Source: CAD feature listing. Evaluate the final solid. Frame: model axes, mm. Face numbers are marked on the shaded views. A direction names the side the tool comes from. Give positions to 0.01 mm unless a question says otherwise; leave off trailing zeros. Write each loop counter-clockwise with the first axis right and the second up, starting at its lowest first coordinate (ties: lowest second). Pieces come first, ordered by that corner, then holes. Notation, with made-up numbers: (-5, 74) -> (34, 74) arc R20 ccw to (34, 96) -> close; hole circle Ø3 at (35.25, 15.25). An arc over 180 degrees is marked (long way). Write item = value, one per line.
from build123d import *

# Parameters (mm, degrees)
SALIENTE_EXTRUIR1_DEPTH = 10
CROQUIS5_R              = 16.5
CORTAR_EXTRUIR4_DEPTH   = 3
CROQUIS4_R              = 1.5
CORTAR_EXTRUIR8_DEPTH   = 126.015998976
CROQUIS6_W              = 60
CROQUIS6_H              = 90.5
SALIENTE_EXTRUIR2_DEPTH = 5
CROQUIS7_R              = 11.25
CROQUIS7_R_2            = 1.5
CORTAR_EXTRUIR9_DEPTH   = 10
SALIENTE_EXTRUIR3_DEPTH = 46
CROQUIS10_W             = 5
CROQUIS10_H             = 5
CORTAR_EXTRUIR11_DEPTH  = 5
CROQUIS11_R             = 1.5
CORTAR_EXTRUIR12_DEPTH  = 168.751304019
CROQUIS13_W             = 43
CROQUIS13_H             = 43
CORTAR_EXTRUIR13_DEPTH  = 2
CROQUIS16_R             = 1
CORTAR_EXTRUIR14_DEPTH  = 10
NERVIO1_REACH           = 159.779
CROQUIS17_WALL_W        = 345.058235512
CROQUIS17_WALL_H        = 10
REDONDEO2_R             = 5
CROQUIS18_W             = 13
CROQUIS18_H             = 12
CORTAR_EXTRUIR15_DEPTH  = 10


with BuildPart() as part:
    # Croquis1 → Saliente-Extruir1 (new body)
    with BuildSketch(Plane.XY):
        with BuildLine():
            Line((-30, -95), (-30, -115))
            Line((-30, -115), (30, -115))
            Line((30, -115), (30, -95))
            ThreePointArc((30, -95), (35.193890367, -54.576427951), (45.544194453, -15.156726282))
            ThreePointArc((45.544194453, -15.156726282), (0, 48), (-45.544194453, -15.156726282))
            ThreePointArc((-45.544194453, -15.156726282), (-35.193890367, -54.576427951), (-30, -95))
        make_face()
    extrude(amount=SALIENTE_EXTRUIR1_DEPTH)

    # Croquis5 → Cortar-Extruir4 (cut)
    with BuildSketch(Plane.XY.offset(10)):
        Circle(CROQUIS5_R)
    extrude(amount=-CORTAR_EXTRUIR4_DEPTH, mode=Mode.SUBTRACT)

    # Croquis4 → Cortar-Extruir8 (cut, through all)
    with BuildSketch(Plane(origin=(0, 0, 10), x_dir=(-1, 0, 0), z_dir=(0, 0, 1))):
        with Locations(Location((0, 12, 0), (0, 0, 180))):
            Circle(CROQUIS4_R)
        with Locations(Location((12, 0, 0), (0, 0, 180))):
            Circle(CROQUIS4_R)
        with Locations(Location((0, -12, 0), (0, 0, 180))):
            Circle(CROQUIS4_R)
        with Locations(Location((-12, 0, 0), (0, 0, 180))):
            Circle(CROQUIS4_R)
    extrude(amount=-CORTAR_EXTRUIR8_DEPTH, mode=Mode.SUBTRACT)

    # Croquis6 → Saliente-Extruir2 (add)
    with BuildSketch(Plane.XZ.offset(115)):
        with Locations((0, 45.25)):
            Rectangle(CROQUIS6_W, CROQUIS6_H)
    extrude(amount=SALIENTE_EXTRUIR2_DEPTH)

    # Croquis7 → Cortar-Extruir9 (cut)
    with BuildSketch(Plane.XZ.offset(120)):
        with Locations(Location((0, 64, 0), (0, 0, 270))):
            Circle(CROQUIS7_R)
        with Locations(Location((-15.5, 79.5, 0), (0, 0, 270))):
            Circle(CROQUIS7_R_2)
        with Locations(Location((15.5, 79.5, 0), (0, 0, 270))):
            Circle(CROQUIS7_R_2)
        with Locations(Location((15.5, 48.5, 0), (0, 0, 270))):
            Circle(CROQUIS7_R_2)
        with Locations(Location((-15.5, 48.5, 0), (0, 0, 270))):
            Circle(CROQUIS7_R_2)
    extrude(amount=-CORTAR_EXTRUIR9_DEPTH, mode=Mode.SUBTRACT)

    # Croquis8 → Saliente-Extruir3 (add)
    with BuildSketch(Plane(origin=(0, -115, 0), x_dir=(1, 0, 0), z_dir=(0, 1, 0))):
        Polygon((-21.5, -42.5), (21.5, -42.5), (21.5, -90.5), (26.5, -90.5), (26.5, -37.5), (-26.5, -37.5), (-26.5, -90.5), (-21.5, -90.5), align=None)
    extrude(amount=SALIENTE_EXTRUIR3_DEPTH)

    # Croquis10 → Cortar-Extruir11 (cut)
    with BuildSketch(Plane.XY.offset(90.5)):
        with Locations((24, -107.5)):
            Rectangle(CROQUIS10_W, CROQUIS10_H)
        with Locations((-24, -107.5)):
            Rectangle(CROQUIS10_W, CROQUIS10_H)
        with Locations((-24, -97.5)):
            Rectangle(CROQUIS10_W, CROQUIS10_H)
        with Locations((24, -97.5)):
            Rectangle(CROQUIS10_W, CROQUIS10_H)
        with Locations((-24, -87.5)):
            Rectangle(CROQUIS10_W, CROQUIS10_H)
        with Locations((24, -87.5)):
            Rectangle(CROQUIS10_W, CROQUIS10_H)
        with Locations((-24, -77.5)):
            Rectangle(CROQUIS10_W, CROQUIS10_H)
        with Locations((24, -77.5)):
            Rectangle(CROQUIS10_W, CROQUIS10_H)
    extrude(amount=-CORTAR_EXTRUIR11_DEPTH, mode=Mode.SUBTRACT)

    # Croquis11 → Cortar-Extruir12 (cut, through all)
    with BuildSketch(Plane.ZY.offset(26.5)):
        with Locations((88, -112.5)):
            Circle(CROQUIS11_R)
        with Locations((88, -72)):
            Circle(CROQUIS11_R)
    extrude(amount=-CORTAR_EXTRUIR12_DEPTH, mode=Mode.SUBTRACT)

    # Croquis13 → Cortar-Extruir13 (cut)
    with BuildSketch(Plane(origin=(0, -115, 0), x_dir=(1, 0, 0), z_dir=(0, 1, 0))):
        with Locations((0, -64)):
            Rectangle(CROQUIS13_W, CROQUIS13_H)
    extrude(amount=-CORTAR_EXTRUIR13_DEPTH, mode=Mode.SUBTRACT)

    # Croquis16 → Cortar-Extruir14 (cut)
    with BuildSketch(Plane.XZ.offset(120)):
        with Locations(Location((-16.25, 64, 0), (0, 0, 270))):
            Circle(CROQUIS16_R)
        with Locations(Location((16.25, 64, 0), (0, 0, 270))):
            Circle(CROQUIS16_R)
        with Locations(Location((-23, 64, 0), (0, 0, 270))):
            Circle(CROQUIS16_R)
        with Locations(Location((23, 64, 0), (0, 0, 270))):
            Circle(CROQUIS16_R)
    extrude(amount=-CORTAR_EXTRUIR14_DEPTH, mode=Mode.SUBTRACT)

    # Croquis17 wall → Nervio1 (add, up to next)
    with BuildSketch(Plane(origin=(0, -69, 23.75), x_dir=(0, 0, -1), z_dir=(0, 1, 0)), mode=Mode.PRIVATE) as nervio1_sk1:
        Rectangle(CROQUIS17_WALL_W, CROQUIS17_WALL_H)
    nervio1_tool1 = extrude(nervio1_sk1.sketch, amount=-NERVIO1_REACH, mode=Mode.PRIVATE) - part.part
    add(nervio1_tool1.solids().sort_by_distance((0, -69, 23.75))[0])

    # Redondeo2
    redondeo2_edges = [part.edges().sort_by_distance(p)[0] for p in [
        (15.75, -115, 37.5),
        (15.75, -69, 37.5),
        (-17.5, -115, 10),
        (-15.75, -69, 37.5),
        (-15.75, -115, 37.5),
        (17.5, -115, 10),
        (5, -69, 23.75),
        (0, -69, 10),
        (5, -115, 23.75),
        (5, -92, 10),
        (-5, -115, 23.75),
        (-5, -92, 10),
        (-5, -69, 23.75),
    ]]
    fillet(redondeo2_edges, radius=REDONDEO2_R - 0.0001)  # a hair under: the kernel refuses the full size

    # Croquis18 → Cortar-Extruir15 (cut)
    with BuildSketch(Plane.ZY.offset(26.5)):
        with Locations((61.5, -75)):
            Rectangle(CROQUIS18_W, CROQUIS18_H)
    extrude(amount=-CORTAR_EXTRUIR15_DEPTH, mode=Mode.SUBTRACT)


solid = part.part
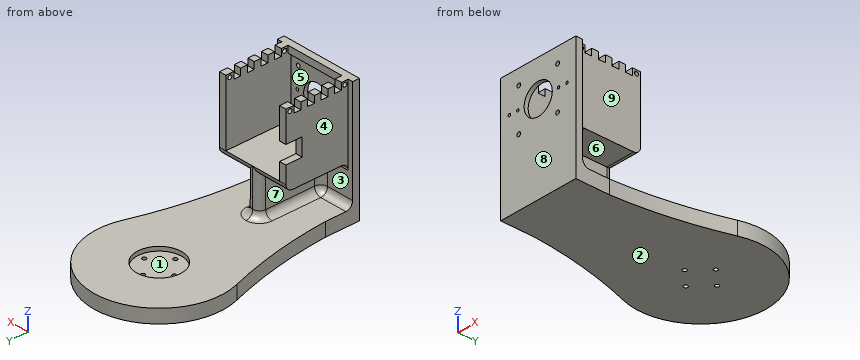
1) Cut plane C-C (y = -92). Return the cut outline in (x, z).
Computed:
outline = (-30.2, 0) -> (30.2, 0) -> (30.2, 10) -> (10, 10) arc R5 cw to (5, 15) -> (5, 37.5) -> (26.5, 37.5) -> (26.5, 90.5) -> (21.5, 90.5) -> (21.5, 42.5) -> (-21.5, 42.5) -> (-21.5, 90.5) -> (-26.5, 90.5) -> (-26.5, 37.5) -> (-5, 37.5) -> (-5, 15) arc R5 cw to (-10, 10) -> (-30.2, 10) -> close
2) Cut plane D-D (x = 34). Return the cut outline in (y, z), then the cut area to 3 significant figures.
Computed:
outline = (-61.07, 0) -> (33.88, 0) -> (33.88, 10) -> (-61.07, 10) -> close
area = 950 mm²
3) Cut plane A-A (z = 73.5). Return the cut outline in (x, y).
Computed:
outline = (-30, -120) -> (-6.03, -120) -> (-6.03, -117) -> (-21.5, -117) -> (-21.5, -69) -> (-26.5, -69) -> (-26.5, -115) -> (-30, -115) -> close; (6.03, -120) -> (30, -120) -> (30, -115) -> (26.5, -115) -> (26.5, -69) -> (21.5, -69) -> (21.5, -117) -> (6.03, -117) -> close
4) Draft query along Z for the marked faces 1, 2, 3 and 4. Return one class per face: pulls with the +Z half, pulls with the -Z half, needs draft (parallel to the pull), parting line crosses it, or undercut.
Computed:
face_1 = pulls with the +Z half
face_2 = pulls with the -Z half
face_3 = undercut
face_4 = needs draft
5) Material intervals for L1, parallel to X at y = -118, z = 64; L2, parallel to Y at x = 0, z = 5; L3, parallel to X at y = -112.75, z = 64, sorted ascending.
Computed:
L1 = -30 to -24, -22 to -17.25, -15.25 to -11.25, 11.25 to 15.25, 17.25 to 22, 24 to 30
L2 = -120 to -13.5, -10.5 to 10.5, 13.5 to 48
L3 = -26.5 to -24, -22 to -21.5, 21.5 to 22, 24 to 26.5
6) Contact query for flat-ended pins moving along their axis: pin 1 (2.5 mm diameter, centred on x = 24, y = -78.5, fed in from +Z); pin 2 (6 mm diameter, centred on x = 25, z = 9.5, fed in from +Y); pin 3 (1 mm diameter, centred on x = 23, z = 64, fed in from -Y). Output: stop coordinate, or through.
Computed:
pin_1 = 85.5
pin_2 = 42.66
pin_3 = -110
7) Access query for the marked faces 5, 6, 7, 8 and 9. Directions: +Z, -Z, +X, -X, +Y, -Y. A direction counts if a zero-diameter tool reaches every point of the face in a straight line with its end or side. Return the directions, or none.
Computed:
face_5 = +Y
face_6 = +X, +Y
face_7 = -X, +Y
face_8 = +Z, -Z, +X, -X, -Y
face_9 = +Z, +X, +Y
